Can you work these out from the model? Positions are in its coordinate system, mm. A direction names the side the tool comes from. Give positions to 0.01 mm unless a question says otherwise; leave off trailing zeros. Order: outer loops, then holes, each group sorted by start corner. A loop starts at its lowest first (then second) coordinate and runs counter-clockwise, first axis right, second up.
Solid Edge part; units mm, degrees
sketch "Sketch1" plane through (0, 0, 0) normal (0, -1, 0) x (1, 0, 0)
  line L0 (105, 85) -> (70, 85)
  line L1 (70, 85) -> (70, 60)
  line L2 (70, 60) -> (65, 60)
  line L3 (65, 60) -> (65, 57)
  line L4 (-115, 57) -> (65, 57)
  line L5 (-115, 0) -> (-115, 57)
  line L6 (-115, 0) -> (105, 0)
  line L7 (105, 0) -> (105, 85)
extrude "Protrusion1" add sketch "Sketch1" along normal mid plane 100
fillet "Round_1" radius 10 1 edges at (105, 0, 85)
sketch "Sketch2" plane through (105, 0, 37.5) normal (1, 0, 0) x (0, 1, 0)
  circle A0 centre (0, -7.5) radius 16
extrude "ExtrudedProtrusion_2" add sketch "Sketch2" along normal blind 5 and the other way blind 121.5371
sketch "Sketch3" plane through (-115, 0, 28.5) normal (-1, 0, 0) x (0, -1, 0)
  circle A0 centre (0, 1.5) radius 16
extrude "ExtrudedProtrusion_4" add sketch "Sketch3" along normal blind 5 and the other way blind 41.3803
sketch "Sketch4" plane through (-25, 0, 57) normal (0, 0, 1) x (0, 1, 0)
  line L0 (-20, 75) -> (-20, -90)
  line L1 (-20, -90) -> (20, -90)
  line L2 (20, -90) -> (20, 75)
  line L3 (20, 75) -> (-20, 75)
extrude "ExtrudedCutout_1" cut sketch "Sketch4" against normal blind 96.6335 and the other way blind 62.4355
hole "Hole_1" at (-120, 0, 30) direction (1, 0, 0) diameter 12 end up to next
hole "Hole_2" at (110, 0, 30) direction (-1, 0, 0) diameter 20 end up to next
sketch "Sketch5" plane through (-5, 0, 0) normal (0, 0, -1) x (1, 0, 0)
  line L0 (-95, 30) -> (70, 30)
  line L1 (70, 30) -> (70, -30)
  line L2 (70, -30) -> (-95, -30)
  line L3 (-95, -30) -> (-95, 30)
extrude "ExtrudedCutout_2" cut sketch "Sketch5" against normal blind 10 and the other way blind 12.0852
sketch "Sketch6" plane through (-5, 0, 0) normal (0, 0, -1) x (1, 0, 0)
  line L0 (-95, 26) -> (70, 26)
  line L1 (70, 26) -> (70, -26)
  line L2 (70, -26) -> (-95, -26)
  line L3 (-95, -26) -> (-95, 26)
extrude "ExtrudedCutout_3" cut sketch "Sketch6" against normal blind 13 and the other way blind 22.4029
hole "Hole_3" at (70, 30, 72.5) direction (1, 0, 0) diameter 4.134 depth 13 thread major 5 thread length 10
hole "Hole1" at (70, -30, 72.5) direction (1, 0, 0) diameter 4.134 depth 13 thread major 5 thread length 10
sketch "Sketch7" plane through (82.5, 0, 85) normal (0, 0, 1) x (0, 1, 0)
  circle A0 centre (0, -7.5) radius 1.5
extrude "ExtrudedCutout_7" cut sketch "Sketch7" against normal up to next and the other way blind 53.7029
chamfer "Chamfer_5" distance 2 angle 45 1 edges at (90, -1.5, 85)
sketch "Sketch8" plane through (-25, 0, 57) normal (0, 0, 1) x (0, -1, 0)
  circle A0 centre (0, -85) radius 1.5
extrude "ExtrudedCutout_8" cut sketch "Sketch8" against normal up to next and the other way blind 4.3365
chamfer "Chamfer_6" distance 2 angle 45 1 edges at (-110, 1.5, 57)
fillet "Round_4" radius 5 1 edges at (105, -16, 30)
fillet "Round_5" radius 5 1 edges at (-115, 16, 30)
sketch "Sketch9" plane through (0, 0, 0) normal (0, 0, 1) x (1, 0, 0)
  line L0 (-5, -90) -> (-25, -90)
  line L1 (-65, -50) -> (-25, -90)
  line L2 (-5, -50) -> (-65, -50)
  line L3 (-5, -50) -> (55, -50)
  line L4 (55, -50) -> (15, -90)
  line L5 (-5, -90) -> (15, -90)
  line L6 (-65, 50) -> (-25, 90)
  line L7 (-5, 90) -> (-25, 90)
  line L8 (-5, 90) -> (15, 90)
  line L9 (55, 50) -> (15, 90)
  line L10 (-5, 50) -> (55, 50)
  line L11 (-5, 50) -> (-65, 50)
extrude "ExtrudedProtrusion_5" add sketch "Sketch9" along normal blind 20
fillet "Round_7" radius 10 4 edges at (-25, -90, 10) (15, -90, 10) (-25, 90, 10) (15, 90, 10)
sketch "Sketch10" plane through (0, 0, 0) normal (0, 0, 1) x (1, 0, 0)
  line L0 (3, 90) -> (3, 77)
  arc A0 (-13, 77) -> (3, 77) centre (-5, 77) ccw
  line L1 (-13, 90) -> (-13, 77)
  line L2 (-18, 90) -> (-13, 90)
  line L3 (-18, 77) -> (-18, 90)
  arc A1 (8, 77) -> (-18, 77) centre (-5, 77) cw
  line L4 (8, 90) -> (8, 77)
  line L5 (3, 90) -> (8, 90)
extrude "ExtrudedProtrusion_7" add sketch "Sketch10" along normal blind 23
sketch "Sketch11" plane through (-5, 79.5, 20) normal (0, 0, 1) x (-1, 0, 0)
  line L0 (-8, -10.5) -> (8, -10.5)
  line L1 (8, -10.5) -> (8, 2.5)
  arc A0 (-8, 2.5) -> (8, 2.5) centre (0, 2.5) cw
  line L2 (-8, -10.5) -> (-8, 2.5)
extrude "Cutout1" cut sketch "Sketch11" against normal through all
mirror "Mirror1" about plane through (0, 0, 0) normal (0, -1, 0) of "ExtrudedProtrusion_7", "Cutout1"
1) Suppose I cut it at D-D (y = -71.5). Please give me the cut outline in (x, z), and give its area (3 significant figures).
2) Which directions (+Z, -Z, +X, -X, +Y, -Y) give clear straight access to the entire face, cutting with the end or side of a thin tool? Please do faces 4 (the face through (-4, -61, 20)), 5 (the face through (-19, -20, 35)), 6 (the face through (68, 1, 60)), 7 (the face through (88, 0, 40)).
3) We'd pull the mould along X, two halves only. Please class faces 1 (the face through (-13, -83, 12)), 2 (the face through (-3, -50, 34)), 3 (the face through (105, 1, 54)): +X half, -X half, draft (parallel to the pull), parting line (faces both ways), or undercut.
4) Suppose I cut it at C-C (x = 78). Please give me the cut outline in (y, z).
5) I'm going to push flat-ended pins straight in: pin 1 Ø1 at (x, y) = (2.5, 34) entering from +Z; pin 2 Ø6.5 at (y, z) = (-82.5, 7.5) entering from -X; pin 3 Ø6.5 at (y, z) = (86, 14.5) entering from +X; pin 4 Ø10 at (x, y) = (-7, -47) entering from -Z. Where does each tip first touch, or does it pass through?
6) If I drill on line 1 (Y direction, x = 76.25, z = 72.5); line 2 (X direction, y = 0, z = 50.75); line 3 (Y direction, x = 79, z = 72), over which ranges is the centre line in solid material (lowest first)?
7) Suppose I cut it at A-A (x = -88.5). Please give me the cut outline in (y, z), and give its area (3 significant figures).
Results:
1. outline: (-43.5, 0) - (-10.81, 0) - (-10.81, 23) - (-16.78, 23) - (-16.78, 20) - (-43.5, 20) - close; (0.81, 0) - (33.5, 0) - (33.5, 20) - (6.78, 20) - (6.78, 23) - (0.81, 23) - close
1. area: 1,340 mm2
2. face 4: +Z
2. face 5: +Z, -Z
2. face 6: +Z, -X, +Y, -Y
2. face 7: +X
3. face 1: undercut
3. face 2: draft
3. face 3: +X half
4. outline: (-50, 0) - (50, 0) - (50, 85) - (-50, 85) - close; hole circle Ø4.13 at (-30, 72.5); hole circle Ø20 at (0, 30); hole circle Ø4.13 at (30, 72.5)
5. pin 1: stops at z = 57
5. pin 2: stops at x = -35.75
5. pin 3: stops at x = 22.25
5. pin 4: stops at z = 0
6. line 1: y = -50 to -32.07, -27.93 to 27.93, 32.07 to 50
6. line 2: x = -115.01 to -111.5, -108.5 to -100, 65 to 88.5, 91.5 to 105.01
6. line 3: y = -50 to -32.01, -27.99 to 27.99, 32.01 to 50
7. outline: (-50, 0) - (-30, 0) - (-30, 10) - (-26, 10) - (-26, 13) - (-20, 13) - (-20, 57) - (-50, 57) - close; (20, 13) - (26, 13) - (26, 10) - (30, 10) - (30, 0) - (50, 0) - (50, 57) - (20, 57) - close
7. area: 3,180 mm2
